from build123d import *

# Parameters (mm, degrees)
SKETCH2_R           = 0.7
BOSS_EXTRUDE2_DEPTH = 30
SKETCH3_R           = 1
BOSS_EXTRUDE3_DEPTH = 0.5


with BuildPart() as part:
    # Sketch1 → Revolve1 (revolve)
    with BuildSketch(Plane.XY):
        with BuildLine():
            Line((0, 3), (0, -3))
            ThreePointArc((0, -3), (3, 0), (0, 3))
        make_face()
    revolve(axis=Axis((0, 3, 0), (0, -1, 0)))

    # Sketch2 → Boss-Extrude2 (add)
    with BuildSketch(Plane.XY):
        with Locations(Location((0, 0, 0), (0, 0, 180))):
            Circle(SKETCH2_R)
    extrude(amount=BOSS_EXTRUDE2_DEPTH)

    # Sketch3 → Boss-Extrude3 (add)
    with BuildSketch(Plane.XY.offset(30)):
        Circle(SKETCH3_R)
    extrude(amount=BOSS_EXTRUDE3_DEPTH)


solid = part.part
Work out the finished part from the listing and answer in its coordinate system (mm). Round coordinates to 2 decimals unless told otherwise and drop trailing zeros. Order: outer loops, then holes, each group sorted by start corner. A loop starts at its lowest first (then second) coordinate and runs counter-clockwise, first axis right, second up. Notation, with made-up numbers: M 14.25,37.5 L 44.25,37.5 A29 cw 44.25,74.5 Z; hole C -27,31.25 d5. An arc over 180 degrees is marked long. Put each result on its own line as item: value. Start each with the question number.
Q1. For a pull along Z with two mould halves and no side action, classify faces 1 (the flat face through (0, 0, 30.5)), 2 (the cylindrical face through (0.7, 0, 16.3)), 3 (the cylindrical face through (-0.217, -0.976, 30.246)) as pulls with the +Z half, pulls with the -Z half, needs draft (parallel to the pull), parting line crosses it, or undercut.
Q2. Section A-A, the plane x = 0 is taken. Write down the section's boundary in (y, z), and give its area (3 significant figures).
Q3. Section D-D, the plane x = 1.75 is taken. Write down the section's boundary in (y, z), and give its area (3 significant figures).
Q4. Straight lines are drawn through the part: L1, parallel to Z at x = -0.1, y = -0.85; L2, parallel to Z at x = -1, y = 1.7; L3, parallel to X at y = 0.4, z = 9.5. For each, find the intervals that lie inside material, in ascending order. Write a range as [from, to].
Q5. Section C-C, the plane z = 20 is taken. Write down the section's boundary in (x, y).
Q6. Flat-ended cylindrical pins translate along their axes: pin 1 (2 mm diameter, centred on x = 1, z = 20, fed in from -Y); pin 2 (3 mm diameter, centred on y = 2.5, z = 15.5, fed in from +X); pin 3 (1.5 mm diameter, centred on x = -2.5, y = -1.5, fed in from -Z); pin 4 (1 mm diameter, centred on y = -1.5, z = 2.5, fed in from -X). Find the tip coordinate at first contact, or state that the pin passes through.
Findings below:
1. face 1: pulls with the +Z half
1. face 2: undercut
1. face 3: needs draft
2. outline: M -1,30 L -0.7,30 L -0.7,2.92 A3 ccw long 0.7,2.92 L 0.7,30 L 1,30 L 1,30.5 L -1,30.5 Z
2. area: 67.1 mm^2
3. outline: C 0,0 d4.87
3. area: 18.7 mm^2
4. L1: z = [-2.88, 2.88], [30, 30.5]
4. L2: z = [-2.26, 2.26]
4. L3: x = [-0.57, 0.57]
5. outline: C 0,0 d1.4
6. pin 1: stops at y = -0.7
6. pin 2: passes through
6. pin 3: stops at z = -2.08
6. pin 4: stops at x = -1.78
